```python
from build123d import *

# Parameters (mm, degrees)
F0_W     = 460
F0_H     = 460
F1_DEPTH = 9


with BuildPart() as f1:
    # F0 (on Top) → F1 (new body)
    with BuildSketch(Plane.XY):
        with Locations((230, 230)):
            Rectangle(F0_W, F0_H)
        with BuildLine():
            Line((252.99375, 61.5), (203.99375, 61.5))
            ThreePointArc((203.99375, 61.5), (190.49375, 75), (203.99375, 88.5))
            Line((203.99375, 88.5), (252.99375, 88.5))
            ThreePointArc((252.99375, 88.5), (266.49375, 75), (252.99375, 61.5))
        make_face(mode=Mode.SUBTRACT)
        with BuildLine():
            ThreePointArc((252.99375, 238.5), (266.49375, 225), (252.99375, 211.5))
            Line((252.99375, 211.5), (203.99375, 211.5))
            ThreePointArc((203.99375, 211.5), (190.49375, 225), (203.99375, 238.5))
            Line((203.99375, 238.5), (252.99375, 238.5))
        make_face(mode=Mode.SUBTRACT)
    extrude(amount=F1_DEPTH)


solid = f1.part
```
CAD build for the part. Positions are in the model's coordinates, mm. A direction names the side the tool comes from. Round coordinates to 2 decimals unless told otherwise and drop trailing zeros. Write each loop counter-clockwise with the first axis right and the second up, starting at its lowest first coordinate (ties: lowest second). Pieces come first, ordered by that corner, then holes. Notation, with made-up numbers: (-20.5, -31.75) - (34.5, -31.75) arc R12 ccw to (34.5, -17.75) - close; hole circle Ø5 at (16.5, -28.75). An arc over 180 degrees is marked (long way). Write item = value, one per line. Start each with the question number.
Q1. Mould opens along Y. For faces 3 (the cylindrical face through (266.49, 225.3, 4.44)), 4 (the cylindrical face through (190.497, 74.703, 4.437)), 5 (the flat face through (227, 284, 0)) say: pulls with the +Y half, pulls with the -Y half, needs draft (parallel to the pull), parting line crosses it, or undercut.
Q2. Which spindle directions (+Z, -Z, +X, -X, +Y, -Y) get a long thin tool onto all of the face, cutting with end or side? Do faces 1 (the flat face through (227, 284, 9)), 2 (the cylindrical face through (266.49, 75.3, 4.44)). Say none if no direction does.
Q3. Probe L1, parallel to X at y = 223.5, z = 3.25; L2, parallel to Y at x = 230.5, z = 0.75; L3, parallel to X at y = 216, z = 3.5. List the from-to ranges inside material, lowest first. Write a range as from..to.
Q4. Band-saw the part on D-D (y = 231). Give the cut face in (x, z), then the cut area to 3 significant figures.
Q5. Band-saw the part on C-C (y = 75). Give the cut face in (x, z), then the cut area to 3 significant figures.
Q6. Band-saw the part on A-A (x = 244.5). Give the cut face in (y, z).
Q7. Band-saw the part on B-B (z = 7). Give the cut face in (x, y).
Answers below:
q1.face_3 = undercut
q1.face_4 = undercut
q1.face_5 = needs draft
q2.face_1 = +Z, +X, -X, +Y, -Y
q2.face_2 = +Z, -Z
q3.L1 = 0..190.58, 266.41..460
q3.L2 = 0..61.5, 88.5..211.5, 238.5..460
q3.L3 = 0..193.93, 263.06..460
q4.outline = (0, 0) - (191.9, 0) - (191.9, 9) - (0, 9) - close; (265.09, 0) - (460, 0) - (460, 9) - (265.09, 9) - close
q4.area = 3,480 mm2
q5.outline = (0, 0) - (190.49, 0) - (190.49, 9) - (0, 9) - close; (266.49, 0) - (460, 0) - (460, 9) - (266.49, 9) - close
q5.area = 3,460 mm2
q6.outline = (0, 0) - (61.5, 0) - (61.5, 9) - (0, 9) - close; (88.5, 0) - (211.5, 0) - (211.5, 9) - (88.5, 9) - close; (238.5, 0) - (460, 0) - (460, 9) - (238.5, 9) - close
q7.outline = (0, 0) - (460, 0) - (460, 460) - (0, 460) - close; hole (203.99, 61.5) - (252.99, 61.5) arc R13.5 ccw to (252.99, 88.5) - (203.99, 88.5) arc R13.5 ccw to start; hole (203.99, 211.5) - (252.99, 211.5) arc R13.5 ccw to (252.99, 238.5) - (203.99, 238.5) arc R13.5 ccw to start
